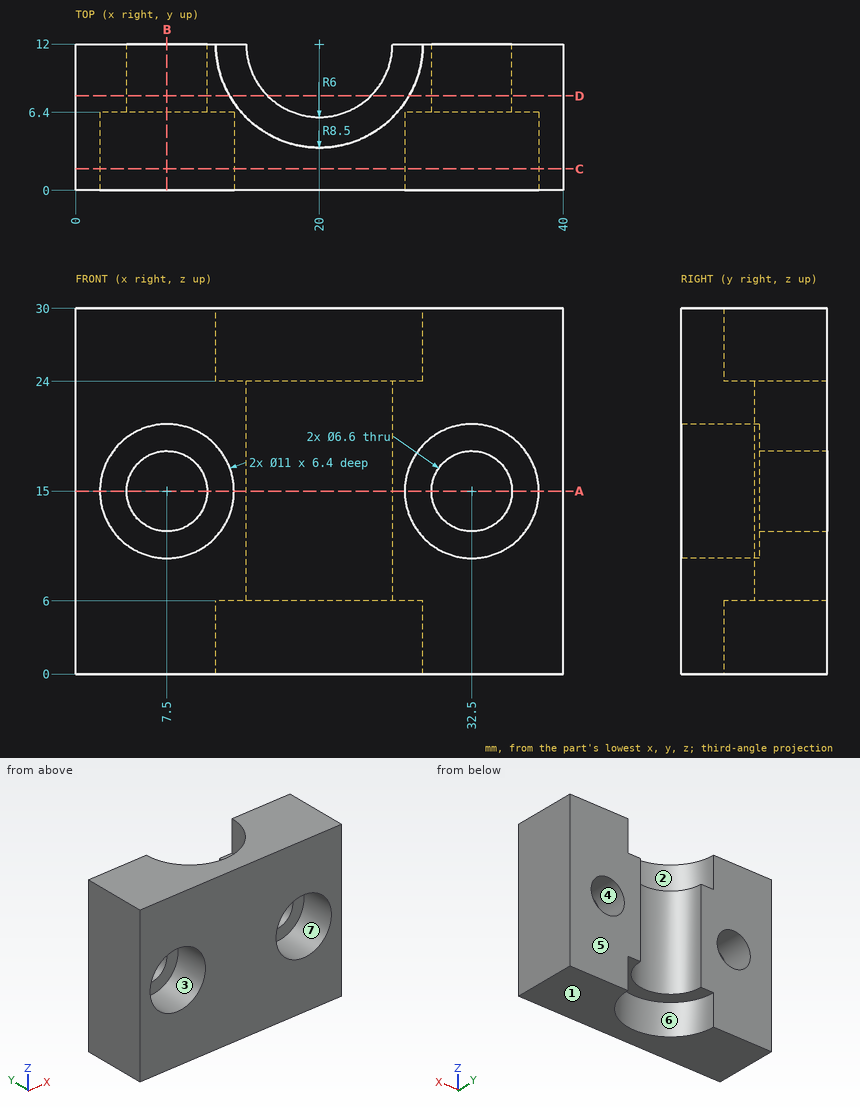
Check sheet for the drawn part. Datum: minimum x, y, z corner. Units: mm. A direction names the side the tool comes from. Round coordinates to 2 decimals unless told otherwise and drop trailing zeros. Order: outer loops, then holes, each group sorted by start corner. A loop starts at its lowest first (then second) coordinate and runs counter-clockwise, first axis right, second up. Notation, with made-up numbers: M 3,43.5 L 49,43.5 A26 cw 49,81.5 Z; hole C 14.25,21.5 d2. An arc over 180 degrees is marked long. Answer in a Markdown table with one row per item.
(1) Section check A-A on z = 15. Record the boundary of the cut face in (x, y), plus the area to 3 significant figures.
Findings:
| item | result |
|---|---|
| outline | M 0,0 L 2,0 L 2,6.4 L 4.2,6.4 L 4.2,12 L 0,12 Z; M 10.8,6.4 L 13,6.4 L 13,0 L 27,0 L 27,6.4 L 29.2,6.4 L 29.2,12 L 26,12 A6 cw 14,12 L 10.8,12 Z; M 35.8,6.4 L 38,6.4 L 38,0 L 40,0 L 40,12 L 35.8,12 Z |
| area | 209 mm^2 |
(2) Section check C-C on y = 1.75. Record the boundary of the cut face in (x, z).
Findings:
| item | result |
|---|---|
| outline | M 0,0 L 40,0 L 40,30 L 0,30 Z; hole C 7.5,15 d11; hole C 32.5,15 d11 |
(3) Draft check along Z on the marked faces 1, 2, 3 and 4. Enter one of: +Z half, -Z half, draft (parallel to the pull), parting line (faces both ways), or undercut.
Findings:
| item | result |
|---|---|
| face 1 | -Z half |
| face 2 | draft |
| face 3 | undercut |
| face 4 | undercut |
(4) Section check D-D on y = 7.75. Record the boundary of the cut face in (x, z), plus the area to 3 significant figures.
Findings:
| item | result |
|---|---|
| outline | M 0,0 L 12.64,0 L 12.64,6 L 15.76,6 L 15.76,24 L 12.64,24 L 12.64,30 L 0,30 Z; M 24.24,6 L 27.36,6 L 27.36,0 L 40,0 L 40,30 L 27.36,30 L 27.36,24 L 24.24,24 Z; hole C 7.5,15 d6.6; hole C 32.5,15 d6.6 |
| area | 802 mm^2 |
(5) Material ranges on line 1 along X through (y, z) = (4, 15.5); line 2 along X through (y, z) = (2.75, 17.5); line 3 along Z through (x, y) = (32.5, 4.5), recorded low to high. Write a range as from..to.
Findings:
| item | result |
|---|---|
| line 1 | x = 0..2.02, 12.98..27.02, 37.98..40 |
| line 2 | x = 0..2.6, 12.4..27.6, 37.4..40 |
| line 3 | z = 0..9.5, 20.5..30 |
(6) Gauge pin test, flat ends, axial feed: pin 1 (9 mm diameter, centred on x = 32.5, z = 15, fed in from -Y); pin 2 (1.5 mm diameter, centred on x = 25.5, z = 26.5, fed in from +Y). Record the tip position at first contact, or that the pin passes through.
Findings:
| item | result |
|---|---|
| pin 1 | stops at y = 6.4 |
| pin 2 | stops at y = 6.24 |
(7) Set-up check for the marked faces 5, 6 and 7: record each of +Z, -Z, +X, -X, +Y, -Y from which the full face is reachable in a straight line by a thin tool's end or side.
Findings:
| item | result |
|---|---|
| face 5 | +Z, -Z, +X, -X, +Y |
| face 6 | -Z, +Y |
| face 7 | -Y |
(8) Section check B-B on x = 7.5. Record the boundary of the cut face in (y, z).
Findings:
| item | result |
|---|---|
| outline | M 0,0 L 12,0 L 12,11.7 L 6.4,11.7 L 6.4,9.5 L 0,9.5 Z; M 0,20.5 L 6.4,20.5 L 6.4,18.3 L 12,18.3 L 12,30 L 0,30 Z |
